from build123d import *

# Parameters (mm, degrees)
BOSS_EXTRU_1_DEPTH      = 6
ESQUISSE2_R             = 1.25
ENL_V_MAT_EXTRU_1_DEPTH = 6


with BuildPart() as part:
    # Esquisse1 → Boss.-Extru.1 (new body)
    with BuildSketch(Plane.XY):
        Polygon((-16.5, 22), (-5, 22), (-5, 16), (5, 16), (5, 22), (16.5, 22), (16.5, -36), (5, -36), (5, -30), (-5, -30), (-5, -36), (-16.5, -36), align=None)
    extrude(amount=BOSS_EXTRU_1_DEPTH)

    # Esquisse2 → Enlèv. mat.-Extru.1 (cut)
    with BuildSketch(Plane.XY.offset(6)):
        with Locations((-10.75, 19)):
            Circle(ESQUISSE2_R)
        with Locations((10.75, 19)):
            Circle(ESQUISSE2_R)
        with Locations((10.75, -19)):
            Circle(ESQUISSE2_R)
        with Locations((-10.75, -19)):
            Circle(ESQUISSE2_R)
    extrude(amount=-ENL_V_MAT_EXTRU_1_DEPTH, mode=Mode.SUBTRACT)


solid = part.part
Can you work these out from the model? Positions are in its coordinate system, mm. A direction names the side the tool comes from. Give positions to 0.01 mm unless a question says otherwise; leave off trailing zeros. Order: outer loops, then holes, each group sorted by start corner. A loop starts at its lowest first (then second) coordinate and runs counter-clockwise, first axis right, second up. Notation, with made-up numbers: M 47.25,-30.5 L 51.25,-30.5 A20 ccw 51.25,-14.5 Z; hole C -20.5,-9 d11. An arc over 180 degrees is marked long. Use one line per item in the form item = value. Start each with the question number.
Item 1: Will this pin go through, and if not, where does the flat tip stop? pin 1 Ø2 at (x, y) = (10.75, 19) entering from -Z.
Item 2: If we section it at A-A (y = -19): Write out the boundary of the cut face in (x, z), then the cut area to 3 significant figures.
Item 3: If we section it at D-D (x = 3.5): Write out the boundary of the cut face in (y, z).
Item 4: If we section it at C-C (x = 10.75): Write out the boundary of the cut face in (y, z), then the cut area to 3 significant figures.
Item 5: If I drill on line 1 along Y through (x, z) = (-10.75, 3.4); line 2 along X through (y, z) = (-33, 2.5); line 3 along Y through (x, z) = (-0.5, 4.9), over which ranges is the centre line in solid material (lowest first)?
Item 6: We'd pull the mould along X, two halves only. Please class faces 4 (the flat face through (0, 16, 3)), 5 (the flat face through (0, -7, 6)), 6 (the flat face through (16.5, -7, 3)), 7 (the flat face through (-16.5, -7, 3)): +X half, -X half, draft (parallel to the pull), parting line (faces both ways), or undercut.
Item 7: If we section it at B-B (z = 2.9): Write out the boundary of the cut face in (x, y), then the cut area to 3 significant figures.
Item 8: For faces 1 (the flat face through (-5, -33, 3)), 2 (the flat face through (-5, 19, 3)), 3 (the flat face through (11, -36, 3)), which set-ups out of +Z, -Z, +X, -X, +Y, -Y let a thin tool reach every point of the face, with its end or its side?
Outcome:
q1.pin_1 = through
q2.outline = M -16.5,0 L -12,0 L -12,6 L -16.5,6 Z; M -9.5,0 L 9.5,0 L 9.5,6 L -9.5,6 Z; M 12,0 L 16.5,0 L 16.5,6 L 12,6 Z
q2.area = 168 mm2
q3.outline = M -30,0 L 16,0 L 16,6 L -30,6 Z
q4.outline = M -36,0 L -20.25,0 L -20.25,6 L -36,6 Z; M -17.75,0 L 17.75,0 L 17.75,6 L -17.75,6 Z; M 20.25,0 L 22,0 L 22,6 L 20.25,6 Z
q4.area = 318 mm2
q5.line_1 = -36 to -20.25, -17.75 to 17.75, 20.25 to 22
q5.line_2 = -16.5 to -5, 5 to 16.5
q5.line_3 = -30 to 16
q6.face_4 = undercut
q6.face_5 = draft
q6.face_6 = +X half
q6.face_7 = -X half
q7.outline = M -16.5,-36 L -5,-36 L -5,-30 L 5,-30 L 5,-36 L 16.5,-36 L 16.5,22 L 5,22 L 5,16 L -5,16 L -5,22 L -16.5,22 Z; hole C -10.75,-19 d2.5; hole C -10.75,19 d2.5; hole C 10.75,-19 d2.5; hole C 10.75,19 d2.5
q7.area = 1,770 mm2
q8.face_1 = +Z, -Z, -Y
q8.face_2 = +Z, -Z, +Y
q8.face_3 = +Z, -Z, +X, -X, -Y
